Input: part model. Units: mm. Frame: model coordinates. A direction names the side the tool comes from. Round coordinates to 2 decimals unless told otherwise and drop trailing zeros. Loops run counter-clockwise (first coordinate to the right, second up) from the corner with the lowest first, then second, coordinate; pieces in that order, holes last.
1) Section A-A, the plane x = 21.25. Return loops of the section in (y, z), and give its area (3 significant figures).
2) Section B-B, the plane y = 12. Return loops of the section in (x, z).
3) Section C-C, the plane z = 22.5. Return loops of the section in (x, y).
4) Section D-D, the plane x = 37.25. Return loops of the section in (y, z).
5) Draft query along Y for faces 1 (the face through (28.4, -26.01, 18.17)), 2 (the face through (28, -31.075, 29)), 3 (the face through (22, 26, 39.67)). Return one class per face: pulls with the +Y half, pulls with the -Y half, needs draft (parallel to the pull), parting line crosses it, or undercut.
6) Access query for faces 4 (the face through (31.707, 26, 30)), 5 (the face through (28.4, 21.99, 44.17)), 6 (the face through (27, 19.425, 15)). Directions: +Z, -Z, +X, -X, +Y, -Y. A direction counts if a zero-diameter tool reaches every point of the face in a straight line with its end or side. Return the directions, or none.
7) Ray query, line 1 along Y through (x, z) = (21.75, 16.67); line 2 along Y through (x, z) = (22.5, 44); line 3 along Y through (x, z) = (28.5, 45). Return the intervals inside material, ascending.
8) First-contact query: pin 1 (4 mm diameter, centred on y = 16, z = 34.5, fed in from -X); pin 2 (8 mm diameter, centred on x = 23, z = 34, fed in from +Y); pin 3 (2.5 mm diameter, centred on y = -26.07, z = 16.67, fed in from -X). Flat tips, straight axial feed; report the tip coordinate or a pass-through.
Autodesk Inventor part; units mm, degrees
ref_plane "YZ Plane" through (0, 0, 0) normal (1, 0, 0) x (0, 1, 0)
ref_plane "XZ Plane" through (0, 0, 0) normal (0, 1, 0) x (-1, 0, 0)
ref_plane "XY Plane" through (0, 0, 0) normal (0, 0, 1) x (1, 0, 0)
ref_plane "Work Plane1" through (13.6834, 18.9252, 14.6894) normal (1, 0, 0) x (0, 1, 0)
sketch "Sketch1" plane through (13.6834, 18.9252, 14.6894) normal (1, 0, 0) x (0, 1, 0)
  circle A0 centre (3, 27.9806) radius 1.5
  circle A1 centre (3, 1.9806) radius 1.5
  circle A2 centre (-45, 1.9806) radius 1.5
  circle A3 centre (-45, 27.9806) radius 1.5
  line L0 (-50, 32.9806) -> (8, 32.9806)
  line L1 (8, 32.9806) -> (8, 24.9805)
  line L2 (8, -3.0194) -> (8, 4.9808)
  line L3 (-50, -3.0194) -> (8, -3.0194)
  line L4 (-50, 0) -> (-50, 32.9806)
  line L5 (-50, -0.0388) -> (-50, -3.0194)
  line L6 (100, 24.9806) -> (0, 24.9806)
  line L7 (0, 22.9806) -> (0, 24.9806)
  line L8 (0, 22.9806) -> (0, 6.9806)
  line L9 (0, 4.9806) -> (0, 6.9806)
  line L10 (0, 4.9806) -> (100, 4.9806)
  line L11 (6, 24.9806) -> (6, 25.4806)
  line L12 (0.5, 30.9806) -> (-42.5, 30.9806)
  line L13 (-48, 25.4806) -> (-48, 4.4806)
  line L14 (-42.5, -1.0194) -> (0.5, -1.0194)
  line L15 (6, 4.4806) -> (6, 4.9806)
  arc A4 (0.5, 27.9806) -> (3, 25.4806) centre (3, 27.9806) ccw
  arc A5 (3, 4.4806) -> (0.5, 1.9806) centre (3, 1.9806) ccw
  arc A6 (-42.5, 1.9806) -> (-45, 4.4806) centre (-45, 1.9806) ccw
  arc A7 (-45, 25.4806) -> (-42.5, 27.9806) centre (-45, 27.9806) ccw
  line L16 (-45, 25.4806) -> (-48, 25.4806)
  line L17 (-42.5, 27.9806) -> (-42.5, 30.9806)
  line L18 (-45, 4.4806) -> (-48, 4.4806)
  line L19 (-42.5, 1.9806) -> (-42.5, -1.0194)
  line L20 (0.5, 1.9806) -> (0.5, -1.0194)
  line L21 (3, 4.4806) -> (6, 4.4806)
  line L22 (0.5, 27.9806) -> (0.5, 30.9806)
  line L23 (3, 25.4806) -> (6, 25.4806)
  circle A8 centre (-45, 1.9806) radius 1.5
  circle A9 centre (-45, 27.9806) radius 1.5
  circle A10 centre (3, 27.9806) radius 1.5
  circle A11 centre (3, 1.9806) radius 1.5
  line L24 (8, 4.9808) -> (8, -3.0194)
  line L25 (-50, -3.0194) -> (8, -3.0194)
  line L26 (-50, -3.0194) -> (-50, 32.9806)
  line L27 (8, 32.9806) -> (-50, 32.9806)
  line L28 (8, 24.9805) -> (8, 32.9806)
  line L29 (8, 24.9805) -> (0, 24.9806)
  line L30 (0, 4.9806) -> (0, 24.9806)
  line L31 (0, 4.9806) -> (8, 4.9808)
  point P0 (-18.9252, -14.6894)
  point P1 (8, 24.9806)
  point P2 (8, 4.9806)
  dimension "d0" = 2
  dimension "d1" = 2
  dimension "d2" = 2
  dimension "d3" = 2
  dimension "d4" = 2
  dimension "d5" = 5
  dimension "d6" = 5
  dimension "d7" = 5
  dimension "d8" = 5
extrude "Extrusion1" add sketch "Sketch1" along normal blind 26.024 contours L0 L1 L6 L11 L23 A4 L22 L12 L17 A7 L16 L13 L18 A6 L19 L14 L20 A5 L21 L15 L10 L2 L3 L5 L26 L4
sketch "Sketch2" plane through (13.6834, -31.0748, 11.67) normal (0, 0, -1) x (-1, 0, 0)
  line L0 (0, 0) -> (-26.024, 0)
  line L1 (-26.024, 0) -> (-29.024, 0)
  line L2 (-29.024, 0) -> (-29.024, 58)
  line L3 (-29.024, 58) -> (-25.5921, 58)
  line L4 (-26.024, 0) -> (-26.024, 58)
  line L5 (-26.024, 0) -> (-26.024, 58)
  point P0 (13.6834, 31.0748)
  dimension "d11" = 3
  dimension "d12" = 58
extrude "Extrusion2" add sketch "Sketch2" against normal up to surface (36 mm away)
sketch "Sketch3" plane through (42.7074, -31.0748, 11.67) normal (1, 0, 0) x (0, 0, -1)
  point P0 (11.67, 31.0748)
sketch "Sketch4" plane through (42.7074, -31.0748, 11.67) normal (1, 0, 0) x (0, 0, -1)
  circle A0 centre (-31, 53) radius 1.5
  circle A1 centre (-5, 53) radius 1.5
  circle A2 centre (-5, 5) radius 1.5
  circle A3 centre (-31, 5) radius 1.5
  point P0 (11.67, 31.0748)
extrude "Extrusion3" cut sketch "Sketch4" against normal through all
sketch "Sketch5" plane through (13.6834, 26.9252, 47.67) normal (0, 1, 0) x (1, 0, 0)
  line L0 (18.024, 10) -> (18.024, 26)
  arc A0 (18.024, 26) -> (16.024, 28) centre (16.024, 26) ccw
  arc A1 (16.024, 8) -> (18.024, 10) centre (16.024, 10) ccw
  line L1 (0.024, 8) -> (16.024, 8)
  line L2 (16.024, 28) -> (0.024, 28)
  line L3 (0, 8) -> (0, 0)
  line L4 (0, 0) -> (29.024, 0)
  line L5 (29.024, 36) -> (29.024, 0)
  line L6 (0, 36) -> (29.024, 36)
  line L7 (0, 36) -> (0, 28)
  line L8 (0, 28) -> (26.024, 28)
  line L9 (26.024, 28) -> (26.024, 8)
  line L10 (0, 8) -> (26.024, 8)
  point P0 (-13.6834, 47.67)
  point P1 (16.024, 8)
extrude "Extrusion4" add sketch "Sketch5" against normal blind 2 contours L0 A0 L8 L9 L10 A1
properties part number "enclosure"
Final values:
1. outline: (-31.07, 11.67) - (26.93, 11.67) - (26.93, 19.67) - (24.93, 19.67) - (24.93, 19.17) - (21.93, 19.17) arc R2.5 ccw to (19.43, 16.67) - (19.43, 13.67) - (-23.57, 13.67) - (-23.57, 16.67) arc R2.5 ccw to (-26.07, 19.17) - (-29.07, 19.17) - (-29.07, 40.17) - (-26.07, 40.17) arc R2.5 ccw to (-23.57, 42.67) - (-23.57, 45.67) - (19.43, 45.67) - (19.43, 42.67) arc R2.5 ccw to (21.93, 40.17) - (24.93, 40.17) - (24.93, 39.67) - (26.93, 39.67) - (26.93, 47.67) - (-31.07, 47.67) - close; hole circle Ø3 at (-26.07, 16.67); hole circle Ø3 at (-26.07, 42.67); hole circle Ø3 at (21.93, 16.67); hole circle Ø3 at (21.93, 42.67)
1. area: 407 mm2
2. outline: (13.68, 11.67) - (42.71, 11.67) - (42.71, 47.67) - (13.68, 47.67) - (13.68, 45.67) - (39.71, 45.67) - (39.71, 13.67) - (13.68, 13.67) - close
3. outline: (13.68, -31.07) - (42.71, -31.07) - (42.71, 26.93) - (31.71, 26.93) - (31.71, 24.93) - (39.71, 24.93) - (39.71, -29.07) - (13.68, -29.07) - close
4. outline: (-31.07, 11.67) - (26.93, 11.67) - (26.93, 47.67) - (-31.07, 47.67) - close; hole (-29.07, 19.17) - (-26.07, 19.17) arc R2.5 cw to (-23.57, 16.67) - (-23.57, 13.67) - (19.43, 13.67) - (19.43, 16.67) arc R2.5 cw to (21.93, 19.17) - (24.93, 19.17) - (24.93, 40.17) - (21.93, 40.17) arc R2.5 cw to (19.43, 42.67) - (19.43, 45.67) - (-23.57, 45.67) - (-23.57, 42.67) arc R2.5 cw to (-26.07, 40.17) - (-29.07, 40.17) - close; hole circle Ø3 at (-26.07, 16.67); hole circle Ø3 at (-26.07, 42.67); hole circle Ø3 at (21.93, 16.67); hole circle Ø3 at (21.93, 42.67)
5. face 1: undercut
5. face 2: pulls with the -Y half
5. face 3: needs draft
6. face 4: -X, +Y
6. face 5: +X, -X
6. face 6: -X
7. line 1: y = -31.07 to -27.57, -24.57 to -23.57, 19.43 to 20.43, 23.43 to 26.93
7. line 2: y = -31.07 to -26.77, -25.38 to -23.57, 19.43 to 21.23, 22.62 to 26.93
7. line 3: y = -31.07 to -23.57, 19.43 to 26.93
8. pin 1: stops at x = 39.71
8. pin 2: stops at y = -29.07
8. pin 3: passes through
